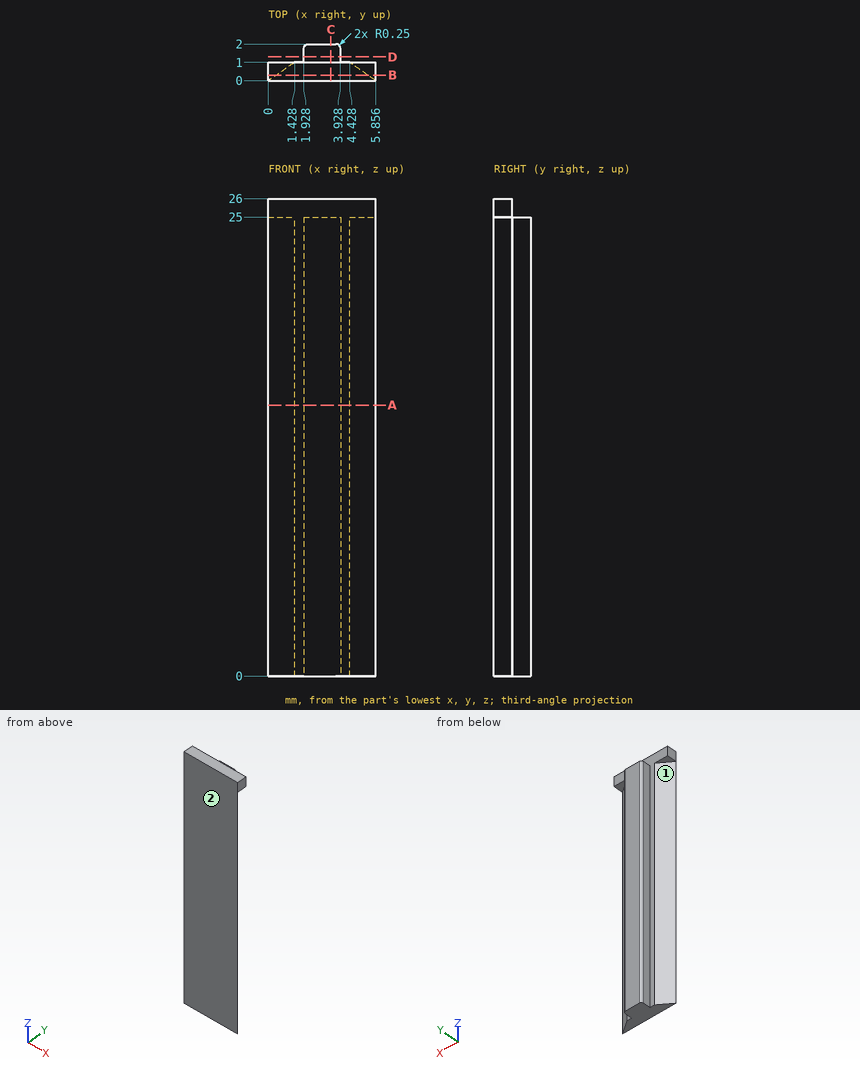
Check sheet for the drawn part. Datum: minimum x, y, z corner. Units: mm. A direction names the side the tool comes from. Give positions to 0.01 mm unless a question says otherwise; leave off trailing zeros. Loops run counter-clockwise (first coordinate to the right, second up) from the corner with the lowest first, then second, coordinate; pieces in that order, holes last. Notation, with made-up numbers: M -26.75,57.25 L 4.25,57.25 A27 cw 4.25,86.25 Z; hole C -38,-7 d8. An arc over 180 degrees is marked long. Answer as CSV lines item,"result".
Item 1: Set-up check for the marked faces 1 and 2: record each of +Z, -Z, +X, -X, +Y, -Y from which the full face is reachable in a straight line by a thin tool's end or side.
Reply:
face 1,"-Z, -X, +Y"
face 2,"+Z, -Z, +X, -X, -Y"
Item 2: Sectioned sample at D-D, the plane y = 1.3. Enter the section's corners in (x, z).
Reply:
outline,"M 1.93,0 L 3.93,0 L 3.93,25 L 1.93,25 Z"
Item 3: Sectioned sample at B-B, the plane y = 0.3. Enter the section's corners in (x, z), then the cut area to 3 significant figures.
Reply:
outline,"M 0,25 L 0.43,25 L 0.43,0 L 5.43,0 L 5.43,25 L 5.86,25 L 5.86,26 L 0,26 Z"
area,"131 mm^2"
Item 4: Sectioned sample at C-C, the plane x = 3.4. Enter the section's corners in (y, z).
Reply:
outline,"M 0,0 L 2,0 L 2,25 L 1,25 L 1,26 L 0,26 Z"
Item 5: Depth check by flat-ended pin: pin 1 Ø2 at (x, z) = (0.5, 20) entering from +Y; pin 2 Ø2 at (x, z) = (3.5, 17) entering from -Y; pin 3 Ø0.8 at (x, y) = (2.5, 1.5) entering from +Z. Enter the tip coordinate at first touch or a pass-through.
Reply:
pin 1,"y = 1"
pin 2,"y = 0"
pin 3,"z = 25"
Item 6: Sectioned sample at A-A, the plane z = 14.75. Enter the section's corners in (x, y).
Reply:
outline,"M 0,0 L 5.86,0 L 4.43,1 L 3.93,1 L 3.93,1.75 A0.25 ccw 3.68,2 L 2.18,2 A0.25 ccw 1.93,1.75 L 1.93,1 L 1.43,1 Z"
Item 7: Scan lines: L1, parallel to Y at x = 2.15, z = 14.5; L2, parallel to X at y = 1.1, z = 2; L3, parallel to Z at x = 3.1, y = 1.15. Record each from-to range of solid material in increasing order.
Reply:
L1,"0 to 2"
L2,"1.93 to 3.93"
L3,"0 to 25"
